Source: CAD feature listing. Evaluate the final solid. Frame: model axes, mm. A direction names the side the tool comes from. Give positions to 0.01 mm unless a question says otherwise; leave off trailing zeros. Order: outer loops, then holes, each group sorted by start corner. A loop starts at its lowest first (then second) coordinate and runs counter-clockwise, first axis right, second up. Notation, with made-up numbers: (-33.5, 68.5) - (-29.5, 68.5) arc R7 ccw to (-29.5, 75.5) - close; hole circle Ø2 at (-4.5, -32). An arc over 180 degrees is marked (long way). Answer as CSV lines item,"result".
```python
from build123d import *

# Parameters (mm, degrees)
SKETCH2_W               = 30
SKETCH2_H               = 80
BOSS_EXTRUDE1_DEPTH     = 3.18
SKETCH4_W               = 10
SKETCH4_H               = 3.12
CUT_EXTRUDE1_DEPTH      = 3.18
MIRROR2_COPY_1_SKETCH_W = 10
MIRROR2_COPY_1_SKETCH_H = 3.12
MIRROR2_COPY_1_DEPTH    = 3.18
SKETCH5_W               = 12.76
SKETCH5_H               = 23.091347567
CUT_EXTRUDE2_DEPTH      = 3.18
SKETCH6_R               = 1
CUT_EXTRUDE3_DEPTH      = 4.18


with BuildPart() as part:
    # Sketch2 → Boss-Extrude1 (new body)
    with BuildSketch(Plane.XY):
        Rectangle(SKETCH2_W, SKETCH2_H)
    extrude(amount=BOSS_EXTRUDE1_DEPTH)

    # Sketch4 → Cut-Extrude1 (cut)
    with BuildSketch(Plane.XY.offset(3.18)):
        with Locations((10, 38.44)):
            Rectangle(SKETCH4_W, SKETCH4_H)
    cut_extrude1 = extrude(amount=-CUT_EXTRUDE1_DEPTH, mode=Mode.SUBTRACT)

    # Mirror1: Cut-Extrude1 across plane
    add(cut_extrude1.mirror(Plane(origin=(0, 0, 0), x_dir=(0, 0, 1), z_dir=(1, 0, 0))), mode=Mode.SUBTRACT)

    # Mirror2: Cut-Extrude1 across plane
    add(cut_extrude1.mirror(Plane.ZX), mode=Mode.SUBTRACT)

    # Mirror2 copy 1 sketch → Mirror2 copy 1 (cut)
    with BuildSketch(Plane(origin=(0, 0, 3.18), x_dir=(-1, 0, 0), z_dir=(0, 0, 1))):
        with Locations((10, 38.44)):
            Rectangle(MIRROR2_COPY_1_SKETCH_W, MIRROR2_COPY_1_SKETCH_H)
    extrude(amount=-MIRROR2_COPY_1_DEPTH, mode=Mode.SUBTRACT)

    # Sketch5 → Cut-Extrude2 (cut)
    with BuildSketch(Plane(origin=(0, 0, 0), x_dir=(-1, 0, 0), z_dir=(0, 0, -1))):
        with Locations((0, 10.179687203)):
            Rectangle(SKETCH5_W, SKETCH5_H)
    extrude(amount=-CUT_EXTRUDE2_DEPTH, mode=Mode.SUBTRACT)

    # Sketch6 → Cut-Extrude3 (cut, through all)
    with BuildSketch(Plane(origin=(0, 0, 0), x_dir=(-1, 0, 0), z_dir=(0, 0, -1))):
        with Locations((0, 24.100360986)):
            Circle(SKETCH6_R)
        with Locations((0, -3.745986581)):
            Circle(SKETCH6_R)
    extrude(amount=-CUT_EXTRUDE3_DEPTH, mode=Mode.SUBTRACT)


solid = part.part
```
(1) Mould query, pull axis Y, two halves, no side actions, for faces 1 (the flat face through (-7, 1, 3.18)), 2 (the flat face through (-6.38, 10, 2)), 3 (the flat face through (0, -40, 2)), 4 (the flat face through (10, 36.88, 2)). Classes: released by +Y, released by -Y, zero draft, split by the parting line, or undercut.
Completed:
face 1,"zero draft"
face 2,"undercut"
face 3,"released by -Y"
face 4,"released by +Y"
(2) Access query for faces 5 (the flat face through (10, -36.88, 2)), 6 (the flat face through (-5, 38, 2)), 7 (the flat face through (-5, -38, 2)), 8 (the flat face through (6.38, 10, 2)), 9 (the flat face through (5, 38, 2)). Directions: +Z, -Z, +X, -X, +Y, -Y. A direction counts if a zero-diameter tool reaches every point of the face in a straight line with its end or side. Return the directions, or none.
Completed:
face 5,"+Z, -Z, +X, -Y"
face 6,"+Z, -Z, -X, +Y"
face 7,"+Z, -Z, -X, -Y"
face 8,"+Z, -Z"
face 9,"+Z, -Z, +X, +Y"
(3) Cut plane B-B (x = 0). Return loops of the section in (y, z).
Completed:
outline,"(-40, 0) - (-4.75, 0) - (-4.75, 3.18) - (-40, 3.18) - close; (-2.75, 0) - (-1.37, 0) - (-1.37, 3.18) - (-2.75, 3.18) - close; (21.73, 0) - (23.1, 0) - (23.1, 3.18) - (21.73, 3.18) - close; (25.1, 0) - (40, 0) - (40, 3.18) - (25.1, 3.18) - close"
(4) Cut plane C-C (z = 0.65). Return loops of the section in (x, y), then the cut area to 3 significant figures.
Completed:
outline,"(-15, -36.88) - (-5, -36.88) - (-5, -40) - (5, -40) - (5, -36.88) - (15, -36.88) - (15, 36.88) - (5, 36.88) - (5, 40) - (-5, 40) - (-5, 36.88) - (-15, 36.88) - close; hole (-6.38, -1.37) - (6.38, -1.37) - (6.38, 21.73) - (-6.38, 21.73) - close; hole circle Ø2 at (0, -3.75); hole circle Ø2 at (0, 24.1)"
area,"1,970 mm²"
(5) Contact query for flat-ended pins moving along their axis: pin 1 (1 mm diameter, centred on x = 8, z = 1, fed in from -Y); pin 2 (1.6 mm diameter, centred on y = -39, z = 1.5, fed in from +X); pin 3 (1.6 mm diameter, centred on y = 39, z = 2, fed in from -X). Output: stop coordinate, or through.
Completed:
pin 1,"y = -36.88"
pin 2,"x = 5"
pin 3,"x = -5"
(6) Cut plane A-A (y = 10.5). Return loops of the section in (x, z), then the cut area to 3 significant figures.
Completed:
outline,"(-15, 0) - (-6.38, 0) - (-6.38, 3.18) - (-15, 3.18) - close; (6.38, 0) - (15, 0) - (15, 3.18) - (6.38, 3.18) - close"
area,"54.8 mm²"
(7) Cut plane D-D (x = -11.25). Return loops of the section in (y, z).
Completed:
outline,"(-36.88, 0) - (36.88, 0) - (36.88, 3.18) - (-36.88, 3.18) - close"
(8) Ray query, line 1 (Y direction, x = 0, z = 1.4); line 2 (Y direction, x = 3.25, z = 0.75); line 3 (Y direction, x = 5.5, z = 0.95). Return the intervals inside material, ascending. Write a range as from..to.
Completed:
line 1,"-40..-4.75, -2.75..-1.37, 21.73..23.1, 25.1..40"
line 2,"-40..-1.37, 21.73..40"
line 3,"-36.88..-1.37, 21.73..36.88"
